CAD build for the part. Positions are in the model's coordinates, mm. A direction names the side the tool comes from. Coordinates: 2 decimals unless noted, no trailing zeros. Order: outer loops, then holes, each group sorted by start corner. A loop starts at its lowest first (then second) coordinate and runs counter-clockwise, first axis right, second up. Notation, with made-up numbers: (19.5, -38.75) - (66.5, -38.75) arc R18 ccw to (66.5, -26.75) - close; hole circle Ø4 at (44.25, 54.25). An arc over 180 degrees is marked (long way). Write each question's results on one line, items separated by ' | '. Start each with the question number.
Q1. Pull direction X, two halves, no side cores. Call faces 1 (the flat face through (-55, -6.35, 22)), 2 (the flat face through (-48.91, 22.18, 6.26)), 3 (the flat face through (12, -12, 38.1)): released by +X, released by -X, zero draft, split by the parting line, or undercut.
Q2. Band-saw the part on D-D, the plane x = -38.5. Write the cut outline in (y, z).
Q3. Band-saw the part on C-C, the plane x = 0. Write the cut outline in (y, z) (3 decimals), then the cut area to 3 significant figures.
Q4. Which spindle directions (+Z, -Z, +X, -X, +Y, -Y) get a long thin tool onto all of the face, cutting with end or side? Do faces 4 (the flat face through (-50, -15, 12.7)), 5 (the flat face through (-88, -7, 25.4)), 6 (the flat face through (-50, 15, 12.7)), 7 (the cylindrical face through (28.55, -1.17, 23.02)). Say none if no direction does.
Q5. Band-saw the part on A-A, the plane y = 0. Write the cut outline in (x, z) (3 decimals), then the cut area to 3 significant figures.
Q6. Pin check, flat tips, straight feed: P1, Ø1.5, axis at x = -26.5, z = 28.5, coming from the -Y side; P2, Ø8, axis at x = -5.5, z = 8.5, coming from the +Y side; P3, Ø1.5, axis at x = -64, y = -12, coming from the +Z side. Stop position of each tip, or through.
Q7. Wall check: probe 1 along Z at (x, y) = (-41.5, -20.5); probe 2 along X at (y, z) = (5.5, 25); probe 3 along Y at (x, z) = (0, 29) (3 decimals). Give the ranges that are in metal, low to high.
Q8. Band-saw the part on B-B, the plane z = 23. Write the cut outline in (x, y) (3 decimals), then the cut area to 3 significant figures.
```python
from build123d import *

# Parameters (mm, degrees)
F0_R          = 9.525
F0_R_2        = 15.875
F1_DEPTH      = 12.7
F2_DEPTH      = 38.1
F3_DEPTH      = 25.4
F5_DEPTH      = 38.1
F7_DEPTH      = 6.35
F7_DEPTH_BACK = 6.35


with BuildPart() as f1:
    # F0 (on Top) → F1 (new body)
    with BuildSketch(Plane.XY):
        with BuildLine():
            ThreePointArc((-79.375, 0), (-79.7098622822, 3.2434155936), (-80.7003221685, 6.35))
            ThreePointArc((-80.7003221685, 6.35), (-86.5549043996, 13.2819779212), (-95.25, 15.875))
            ThreePointArc((-95.25, 15.875), (-111.125, 0), (-95.25, -15.875))
            ThreePointArc((-95.25, -15.875), (-86.5549043996, -13.2819779212), (-80.7003221685, -6.35))
            ThreePointArc((-80.7003221685, -6.35), (-79.7098622822, -3.2434155936), (-79.375, 0))
        make_face()
        with Locations((-95.25, 0)):
            Circle(F0_R, mode=Mode.SUBTRACT)
        with BuildLine():
            ThreePointArc((-27.86051193, -6.35), (-28.575, 0), (-27.86051193, 6.35))
            Line((-27.86051193, 6.35), (-80.7003221685, 6.35))
            ThreePointArc((-80.7003221685, 6.35), (-79.7098622822, 3.2434155936), (-79.375, 0))
            ThreePointArc((-79.375, 0), (-79.7098622822, -3.2434155936), (-80.7003221685, -6.35))
            Line((-80.7003221685, -6.35), (-27.86051193, -6.35))
        make_face()
        with BuildLine():
            Line((-80.7003221685, 6.35), (-27.86051193, 6.35))
            ThreePointArc((-27.86051193, 6.35), (-19.2885651774, 21.0827388732), (-3.8535043435, 28.3139740989))
            Line((-3.8535043435, 28.3139740989), (-95.25, 15.875))
            ThreePointArc((-95.25, 15.875), (-86.5549043996, 13.2819779212), (-80.7003221685, 6.35))
        make_face()
        with BuildLine():
            ThreePointArc((-3.8535043435, -28.3139740989), (-19.2885651774, -21.0827388732), (-27.86051193, -6.35))
            Line((-27.86051193, -6.35), (-80.7003221685, -6.35))
            ThreePointArc((-80.7003221685, -6.35), (-86.5549043996, -13.2819779212), (-95.25, -15.875))
            Line((-95.25, -15.875), (-3.8535043435, -28.3139740989))
        make_face()
        with BuildLine():
            ThreePointArc((-3.8535043435, 28.3139740989), (-19.2885651774, 21.0827388732), (-27.86051193, 6.35))
            ThreePointArc((-27.86051193, 6.35), (-28.575, 0), (-27.86051193, -6.35))
            ThreePointArc((-27.86051193, -6.35), (-19.2885651774, -21.0827388732), (-3.8535043435, -28.3139740989))
            ThreePointArc((-3.8535043435, -28.3139740989), (18.7938385965, -21.5249217376), (28.575, 0))
            ThreePointArc((28.575, 0), (18.7938385965, 21.5249217375), (-3.8535043435, 28.3139740989))
        make_face()
        Circle(F0_R_2, mode=Mode.SUBTRACT)
    extrude(amount=F1_DEPTH)

    # F0 (on Top) → F2 (join)
    with BuildSketch(Plane.XY):
        with BuildLine():
            ThreePointArc((-3.8535043435, 28.3139740989), (-19.2885651774, 21.0827388732), (-27.86051193, 6.35))
            ThreePointArc((-27.86051193, 6.35), (-28.575, 0), (-27.86051193, -6.35))
            ThreePointArc((-27.86051193, -6.35), (-19.2885651774, -21.0827388732), (-3.8535043435, -28.3139740989))
            ThreePointArc((-3.8535043435, -28.3139740989), (18.7938385965, -21.5249217376), (28.575, 0))
            ThreePointArc((28.575, 0), (18.7938385965, 21.5249217375), (-3.8535043435, 28.3139740989))
        make_face()
        Circle(F0_R_2, mode=Mode.SUBTRACT)
    extrude(amount=F2_DEPTH)

    # F0 (on Top) → F3 (join)
    with BuildSketch(Plane.XY):
        with BuildLine():
            ThreePointArc((-79.375, 0), (-79.7098622822, 3.2434155936), (-80.7003221685, 6.35))
            ThreePointArc((-80.7003221685, 6.35), (-86.5549043996, 13.2819779212), (-95.25, 15.875))
            ThreePointArc((-95.25, 15.875), (-111.125, 0), (-95.25, -15.875))
            ThreePointArc((-95.25, -15.875), (-86.5549043996, -13.2819779212), (-80.7003221685, -6.35))
            ThreePointArc((-80.7003221685, -6.35), (-79.7098622822, -3.2434155936), (-79.375, 0))
        make_face()
        with Locations((-95.25, 0)):
            Circle(F0_R, mode=Mode.SUBTRACT)
    extrude(amount=F3_DEPTH)

    # F0 (on Top) → F5 (join, through all)
    with BuildSketch(Plane.XY):
        with BuildLine():
            ThreePointArc((-27.86051193, -6.35), (-28.575, 0), (-27.86051193, 6.35))
            Line((-27.86051193, 6.35), (-80.7003221685, 6.35))
            ThreePointArc((-80.7003221685, 6.35), (-79.7098622822, 3.2434155936), (-79.375, 0))
            ThreePointArc((-79.375, 0), (-79.7098622822, -3.2434155936), (-80.7003221685, -6.35))
            Line((-80.7003221685, -6.35), (-27.86051193, -6.35))
        make_face()
    extrude(amount=F5_DEPTH)

    # F6 (on Front) → F7 (cut, two sides)
    with BuildSketch(Plane.XZ) as f7_sk:
        Polygon((-80.7003221685, 25.4), (-79.375, 25.4), (-28.575, 38.1), (-80.7003221685, 38.1), align=None)
    extrude(amount=-F7_DEPTH, mode=Mode.SUBTRACT)
    extrude(f7_sk.sketch, amount=F7_DEPTH_BACK, mode=Mode.SUBTRACT)


solid = f1.part
```
Results below:
1) face 1: undercut | face 2: released by -X | face 3: zero draft
2) outline: (-23.6, 0) - (23.6, 0) - (23.6, 12.7) - (6.35, 12.7) - (6.35, 35.62) - (-6.35, 35.62) - (-6.35, 12.7) - (-23.6, 12.7) - close
3) outline: (-28.575, 0) - (-15.875, 0) - (-15.875, 38.1) - (-28.575, 38.1) - close; (15.875, 0) - (28.575, 0) - (28.575, 38.1) - (15.875, 38.1) - close | area: 968 mm²
4) face 4: +Z, -Y | face 5: +Z, -X, +Y, -Y | face 6: +Z, +Y | face 7: +Z
5) outline: (-111.125, 0) - (-104.775, 0) - (-104.775, 25.4) - (-111.125, 25.4) - close; (-85.725, 0) - (-15.875, 0) - (-15.875, 38.1) - (-28.575, 38.1) - (-79.375, 25.4) - (-85.725, 25.4) - close; (15.875, 0) - (28.575, 0) - (28.575, 38.1) - (15.875, 38.1) - close | area: 2,900 mm²
6) P1: stops at y = -12.39 | P2: stops at y = 28.54 | P3: stops at z = 12.7
7) probe 1: z = 0 to 12.7 | probe 2: x = -110.14 to -103.03, -87.47 to -14.89, 14.89 to 28.04 | probe 3: y = -28.575 to -15.875, 15.875 to 28.575
8) outline: (-80.7, -6.35) - (-27.861, -6.35) arc R28.575 ccw (long way) to (-27.861, 6.35) - (-80.7, 6.35) arc R15.875 ccw (long way) to start; hole circle Ø19.05 at (-95.25, 0); hole circle Ø31.75 at (0, 0) | area: 2,930 mm²
